from build123d import *

# Parameters (mm, degrees)
SKETCH2_W           = 18.82
SKETCH2_H           = 15.67
BOSS_EXTRUDE1_DEPTH = 3.805
SKETCH3_R           = 3
BOSS_EXTRUDE2_DEPTH = 1.49
SKETCH4_R           = 1.5
BOSS_EXTRUDE3_DEPTH = 2.7


with BuildPart() as part:
    # Sketch2 → Boss-Extrude1 (new, symmetric)
    with BuildSketch(Plane.XY):
        Rectangle(SKETCH2_W, SKETCH2_H)
    extrude(amount=BOSS_EXTRUDE1_DEPTH, both=True)

    # Sketch3 → Boss-Extrude2 (add)
    with BuildSketch(Plane(origin=(0, 7.835, 0), x_dir=(1, 0, 0), z_dir=(0, 1, 0))):
        with Locations((-4.98, 0)):
            Circle(SKETCH3_R)
    extrude(amount=BOSS_EXTRUDE2_DEPTH)

    # Sketch4 → Boss-Extrude3 (add)
    with BuildSketch(Plane(origin=(0, 9.325, 0), x_dir=(1, 0, 0), z_dir=(0, 1, 0))):
        with Locations((-4.98, 0)):
            Circle(SKETCH4_R)
    extrude(amount=BOSS_EXTRUDE3_DEPTH)


solid = part.part
Check sheet for the modelled part. Datum: model origin and axes. Units: mm. A direction names the side the tool comes from. Round coordinates to 2 decimals unless told otherwise and drop trailing zeros. Order: outer loops, then holes, each group sorted by start corner. A loop starts at its lowest first (then second) coordinate and runs counter-clockwise, first axis right, second up.
Q1. Scan lines: L1, parallel to Y at x = 5.75, z = 1.5 (3 decimals); L2, parallel to Y at x = -5, z = 2.25 (3 decimals); L3, parallel to Z at x = -4.5, y = 10.5. Record each from-to range of solid material in increasing order.
Filled sheet:
L1: y = -7.835 to 7.835
L2: y = -7.835 to 9.325
L3: z = -1.42 to 1.42
Q2. Cross-section at B-B, the plane x = -4.98. Enter the section's corners in (y, z) (3 decimals).
Filled sheet:
outline: (-7.835, -3.805) - (7.835, -3.805) - (7.835, -3) - (9.325, -3) - (9.325, -1.5) - (12.025, -1.5) - (12.025, 1.5) - (9.325, 1.5) - (9.325, 3) - (7.835, 3) - (7.835, 3.805) - (-7.835, 3.805) - close
Q3. Cross-section at C-C, the plane x = 5. Enter the section's corners in (y, z) (3 decimals).
Filled sheet:
outline: (-7.835, -3.805) - (7.835, -3.805) - (7.835, 3.805) - (-7.835, 3.805) - close
Q4. Depth check by flat-ended pin: P1, Ø2.5, axis at x = 4.5, z = 1.5, coming from the +Y side (3 decimals). Enter the tip coordinate at first touch or a pass-through.
Filled sheet:
P1: stops at y = 7.835
Q5. Set-up check for faces 1 (the face through (0, 0, -3.805)), 2 (the face through (-3.55, 10.66, -0.45)): record each of +Z, -Z, +X, -X, +Y, -Y from which the full face is reachable in a straight line by a thin tool's end or side.
Filled sheet:
face 1: -Z, +X, -X, +Y, -Y
face 2: +Y
Q6. Cross-section at D-D, the plane x = -7. Enter the section's corners in (y, z) (3 decimals).
Filled sheet:
outline: (-7.835, -3.805) - (7.835, -3.805) - (7.835, -2.218) - (9.325, -2.218) - (9.325, 2.218) - (7.835, 2.218) - (7.835, 3.805) - (-7.835, 3.805) - close
Q7. Cross-section at A-A, the plane z = 0. Enter the section's corners in (x, y) (3 decimals).
Filled sheet:
outline: (-9.41, -7.835) - (9.41, -7.835) - (9.41, 7.835) - (-1.98, 7.835) - (-1.98, 9.325) - (-3.48, 9.325) - (-3.48, 12.025) - (-6.48, 12.025) - (-6.48, 9.325) - (-7.98, 9.325) - (-7.98, 7.835) - (-9.41, 7.835) - close
